Print and shaded views of the part. All mm, measured from the part's lowest x, y and z. Round coordinates to 2 decimals unless told otherwise and drop trailing zeros. Loops run counter-clockwise (first coordinate to the right, second up) from the corner with the lowest first, then second, coordinate; pieces in that order, holes last. Notation, with made-up numbers: (-22.75, -5) - (8.25, -5) arc R7 ccw to (8.25, 7) - close; hole circle Ø5 at (-37, 86). An arc over 180 degrees is marked (long way). Use one line per item in the form item = value.
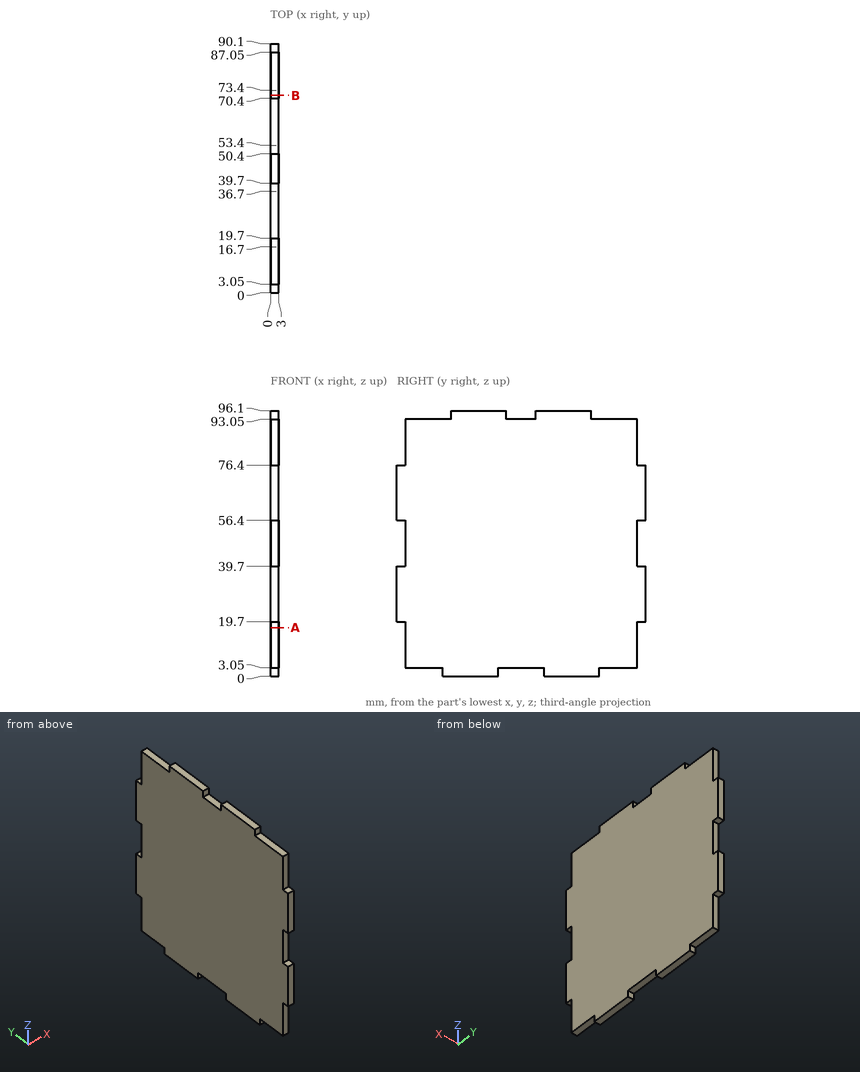
1. Flat gauge pins, fed straight in: pin 1 (1.5 mm diameter, centred on x = 1, y = 1, fed in from -Z); pin 2 (0.9 mm diameter, centred on x = 2, y = 15, fed in from +Z); pin 3 (0.9 mm diameter, centred on x = 2, z = 94, fed in from -Y); pin 4 (6 mm diameter, centred on y = 32.5, z = 80.5, fed in from -X). Where does each tip first touch, or does it go through?
Geometry check:
pin_1 = 19.7
pin_2 = 93.05
pin_3 = 19.7
pin_4 = 0
2. Cut at B-B, the plane y = 71.5. Give the cut face in (x, z), plus the area to 3 significant figures.
Geometry check:
outline = (0, 0) - (3, 0) - (3, 93.05) - (0, 93.05) - close
area = 279 mm^2
3. Wall check: probe 1 along Y at (x, z) = (2.85, 16.5); probe 2 along Z at (x, y) = (2.7, 39); probe 3 along Z at (x, y) = (1.9, 9). Give the ranges that are in metal, low to high.
Geometry check:
probe_1 = 3.05 to 87.05
probe_2 = 3.05 to 96.1
probe_3 = 3.05 to 93.05
4. Cut at A-A, the plane z = 17.5. Give the cut face in (x, y), plus the area to 3 significant figures.
Geometry check:
outline = (0, 3.05) - (3, 3.05) - (3, 87.05) - (0, 87.05) - close
area = 252 mm^2
